Geometry: final body of the model. Coordinates: model frame, mm. Coordinates: 2 decimals unless noted, no trailing zeros. Order: outer loops, then holes, each group sorted by start corner. A loop starts at its lowest first (then second) coordinate and runs counter-clockwise, first axis right, second up. Notation, with made-up numbers: M 85,-20.5 L 110,-20.5 A26 ccw 110,12.5 Z; hole C 64,28.5 d11. An arc over 180 degrees is marked long. One line per question, with ' | ' between items.
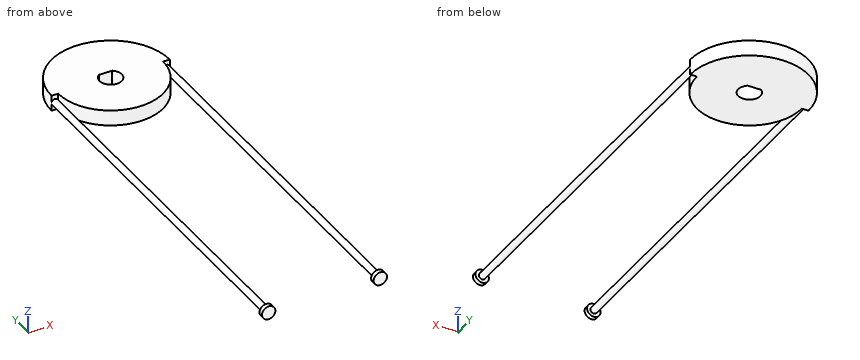
from build123d import *

# Parameters (mm, degrees)
CUT_EXTRUDE1_DEPTH  = 9
CUT_EXTRUDE2_START  = -7
CUT_EXTRUDE2_DEPTH  = 7
SKETCH6_R           = 1.5
BOSS_EXTRUDE1_DEPTH = 170
SKETCH7_R           = 3
BOSS_EXTRUDE2_DEPTH = 2


with BuildPart() as part:
    # Sketch2 → Revolve1 (revolve)
    with BuildSketch(Plane(origin=(0, 0, 0), x_dir=(0, 0, -1), z_dir=(1, 0, 0)), mode=Mode.PRIVATE) as revolve1_sk:
        Polygon((-3.561959221, 0), (3.438040779, 0), (3.438040779, 26.5), (1.438040779, 26.5), (-1.561959221, 26.5), (-3.561959221, 26.5), align=None)
    revolve(revolve1_sk.sketch.rotate(Axis((0, 0, 3.561959221), (0, 0, -1)), 90), axis=Axis((0, 0, 3.561959221), (0, 0, -1)))

    # Sketch3 → Cut-Extrude1 (cut)
    with BuildSketch(Plane(origin=(0, 0, -3.438040779), x_dir=(-1, 0, 0), z_dir=(0, 0, -1))):
        with BuildLine():
            Line((-2.95661762, 4.03217215), (3.043032331, 3.967361117))
            ThreePointArc((3.043032331, 3.967361117), (-0.054009195, -4.999708292), (-2.95661762, 4.03217215))
        make_face()
    extrude(amount=-CUT_EXTRUDE1_DEPTH, mode=Mode.SUBTRACT)

    # Sketch5 → Cut-Extrude2 (cut)
    with BuildSketch(Plane(origin=(0, 0, -3.438040779), x_dir=(-1, 0, 0), z_dir=(0, 0, -1)).offset(CUT_EXTRUDE2_START)):
        with BuildLine():
            Line((-26.5, 0), (-23.5, 0))
            ThreePointArc((-23.5, 0), (0, -23.5), (23.5, 0))
            Line((23.5, 0), (26.5, 0))
            ThreePointArc((26.5, 0), (0, -26.5), (-26.5, 0))
        make_face()
    extrude(amount=CUT_EXTRUDE2_DEPTH, mode=Mode.SUBTRACT)

    # Sketch6 → Boss-Extrude1 (add)
    with BuildSketch(Plane.XZ):
        with Locations(Location((25, 0.061959221, 0), (0, 0, 180))):
            Circle(SKETCH6_R)
        with Locations(Location((-25, 0.061959221, 0), (0, 0, 180))):
            Circle(SKETCH6_R)
    extrude(amount=BOSS_EXTRUDE1_DEPTH)

    # Sketch7 → Boss-Extrude2 (add)
    with BuildSketch(Plane.XZ.offset(170)):
        with Locations(Location((25, 0.061959221, 0), (0, 0, 270))):
            Circle(SKETCH7_R)
        with Locations(Location((-25, 0.061959221, 0), (0, 0, 270))):
            Circle(SKETCH7_R)
    extrude(amount=BOSS_EXTRUDE2_DEPTH)


solid = part.part
1. Section C-C, the plane x = -8.5. Output: boundary loops of the cut face in (y, z), and give its area (3 significant figures).
Response values:
outline: M -21.91,-3.44 L 25.1,-3.44 L 25.1,3.56 L -21.91,3.56 Z | area: 329 mm^2
2. Pin query (flat end, axial travel): P1, Ø1.8, axis at x = 24.5, z = -1, coming from the +Y side; P2, Ø5, axis at x = 20.5, y = -32.5, coming from the -Z side; P3, Ø3, axis at y = -61.5, z = -1.5, coming from the +X side; P4, Ø1.5, axis at x = -9.5, z = -0.5, coming from the -Y side. Return the tip coordinate at first contact, or that it passes through.
Response values:
P1: stops at y = 12.05 | P2: passes through | P3: stops at x = 26.5 | P4: stops at y = -21.81
3. Material intervals for line 1 (Y direction, x = 0, z = 0.5); line 2 (Y direction, x = 14.5, z = -2); line 3 (Y direction, x = 10, z = -1.25), sorted ascending. Write a range as [from, to].
Response values:
line 1: y = [-23.5, -5], [4, 26.5] | line 2: y = [-18.49, 22.18] | line 3: y = [-21.27, 24.54]
4. Section B-B, the plane y = -57.5. Output: boundary loops of the cut face in (x, z).
Response values:
outline: C -25,0.06 d3; C 25,0.06 d3
5. Section A-A, the plane x = 0. Output: boundary loops of the cut face in (y, z), and give its area (3 significant figures).
Response values:
outline: M -23.5,-3.44 L -5,-3.44 L -5,3.56 L -23.5,3.56 Z; M 4,-3.44 L 26.5,-3.44 L 26.5,3.56 L 4,3.56 Z | area: 287 mm^2
